Input: part model. Units: mm. Frame: model coordinates. A direction names the side the tool comes from. Give positions to 0.01 mm unless a question says otherwise; leave off trailing zeros. Write each loop counter-clockwise with the first axis right and the second up, starting at its lowest first coordinate (ties: lowest second). Pieces come first, ordered by that corner, then holes. Notation, with made-up numbers: (74, 76) -> (132, 76) arc R14 cw to (132, 94) -> close; hole circle Ø8 at (57, 60). An arc over 180 degrees is marked (long way). Return JSON: item names as keys, results as strings. Group by question number.
Item 1: Section C-C, the plane x = -25. Return loops of the section in (y, z), then the cut area to 3 significant figures.
Item 2: Section A-A, the plane z = 0. Return loops of the section in (x, y), then the cut area to 3 significant figures.
Item 3: Mould query, pull axis Z, two halves, no side actions, for faces 3 (the face through (24.033, -25.028, -3.286)), 4 (the face through (10.85, -1.34, 2.11)), 5 (the face through (-46.21, 5, 0)). Classes: released by +Z, released by -Z, zero draft, split by the parting line, or undercut.
Item 4: Line query: line 1 (Z direction, x = -28, y = 0); line 2 (Z direction, x = 3, y = 0). Output: solid intervals per line, ascending. Write a range as [from, to].
Item 5: Pin query (flat end, axial travel): P1, Ø10, axis at y = 0, z = 0, coming from the -X side; P2, Ø2, axis at x = -28.5, z = 5.5, coming from the +Y side; P3, Ø8, axis at x = 6.5, y = 8, coming from the +Z side; P4, Ø10, axis at x = -20, z = -4, coming from the -Y side. Return the tip coordinate at first contact, or that it passes through.
Item 6: Set-up query: faces 1 (the face through (-11.7, -3.755, 11.923)), 2 (the face through (33.72, -1.32, -29.97)). Return all of +Z, -Z, +X, -X, +Y, -Y with unobstructed straight access to the full face (end or side cutting, diameter ignored); none if empty.
from build123d import *

# Parameters (mm, degrees)
F3_D     = 8.8
F3_DEPTH = 28.75
F3_TIP   = 2.6437867237
F5_D     = 5


# Not quite as in the source:
# - a feature names something its author has since deleted; it is built from what else it names


with BuildPart() as f1:
    # F0 (on Front) → F1 (revolve)
    with BuildSketch(Plane.XZ):
        Polygon((23.7903209624, 12.5), (-46.2096790376, 12.5), (-46.2096790376, 0), (38.7903209624, 0), (38.7903209624, 30), (28.7903209624, 30), (23.7903209624, 25), align=None)
    revolve(axis=Axis((-0.8820928633, 0, 0), (1, 0, 0)))

    # F3
    with Locations(Plane(origin=(-46.2096790376, 0, 0), x_dir=(0, -1, 0), z_dir=(-1, 0, 0))):
        with Locations((0, 0)):
            Hole(F3_D / 2, depth=F3_DEPTH)
            with Locations((0, 0, -(F3_DEPTH + F3_TIP / 2))):  # 118° drill point
                Cone(0, F3_D / 2, F3_TIP, mode=Mode.SUBTRACT)

    # F5 (through all)
    with Locations(Plane.YZ.offset(38.7903209624)):
        with Locations((0, 0)):
            Hole(F5_D / 2)


solid = f1.part
Answer below:
{
 "1": {"outline": "circle Ø25 at (0, 0); hole circle Ø8.8 at (0, 0)", "area": "430 mm2"},
 "2": {"outline": "(-46.21, -12.5) -> (23.79, -12.5) -> (23.79, -25) -> (28.79, -30) -> (38.79, -30) -> (38.79, -2.5) -> (-16.32, -2.5) -> (-17.46, -4.4) -> (-46.21, -4.4) -> close; (-46.21, 4.4) -> (-17.46, 4.4) -> (-16.32, 2.5) -> (38.79, 2.5) -> (38.79, 30) -> (28.79, 30) -> (23.79, 25) -> (23.79, 12.5) -> (-46.21, 12.5) -> close", "area": "2,090 mm2"},
 "3": {"face 3": "split by the parting line", "face 4": "undercut", "face 5": "zero draft"},
 "4": {"line 1": "z = [-12.5, -4.4], [4.4, 12.5]", "line 2": "z = [-12.5, -2.5], [2.5, 12.5]"},
 "5": {"P1": "stops at x = -46.21", "P2": "stops at y = 11.66", "P3": "stops at z = 11.84", "P4": "stops at y = -12.5"},
 "6": {"face 1": "-X", "face 2": "+X, -X"}
}
